Design review of the part built by this model. Coordinates are the model's own, in mm. A direction names the side the tool comes from. Coordinates: 2 decimals unless noted, no trailing zeros. Write each loop counter-clockwise with the first axis right and the second up, starting at its lowest first coordinate (ties: lowest second). Pieces come first, ordered by that corner, then holes.
```python
from build123d import *

# Parameters (mm, degrees)
SKETCH_1_R           = 23
EXTRUDE_1_DEPTH      = 26
SKETCH_7_R           = 23
SKETCH_7_R_2         = 15
CUT_EXTRUDE_5_DEPTH  = 8
SKETCH_8_R           = 9.5
CUT_EXTRUDE_6_DEPTH  = 6
SKETCH_9_R           = 3
CUT_EXTRUDE_7_DEPTH  = 24.5
SKETCH_10_R          = 20
CUT_EXTRUDE_8_DEPTH  = 10
CUT_EXTRUDE_START    = -6
SKETCH_11_R          = 9.5
CUT_EXTRUDE_10_DEPTH = 6


with BuildPart() as part:
    # 스케치1 → 보스-돌출1 (new body)
    with BuildSketch(Plane(origin=(0, 0, 0), x_dir=(1, 0, 0), z_dir=(0, 1, 0))):
        with Locations(Location((0, 0, 0), (0, 0, 90))):
            Circle(SKETCH_1_R)
    extrude(amount=EXTRUDE_1_DEPTH)

    # 스케치7 → 컷-돌출5 (cut)
    with BuildSketch(Plane(origin=(0, 0, 0), x_dir=(-1, 0, 0), z_dir=(0, -1, 0))):
        with Locations(Location((0, 0, 0), (0, 0, 90))):
            Circle(SKETCH_7_R)
        with Locations(Location((0, 0, 0), (0, 0, 90))):
            Circle(SKETCH_7_R_2, mode=Mode.SUBTRACT)
    extrude(amount=-CUT_EXTRUDE_5_DEPTH, mode=Mode.SUBTRACT)

    # 스케치8 → 컷-돌출6 (cut)
    with BuildSketch(Plane.XZ):
        with Locations(Location((0, 0, 0), (0, 0, 270))):
            Circle(SKETCH_8_R)
    extrude(amount=-CUT_EXTRUDE_6_DEPTH, mode=Mode.SUBTRACT)

    # 스케치9 → 컷-돌출7 (cut)
    with BuildSketch(Plane(origin=(0, 26, 0), x_dir=(1, 0, 0), z_dir=(0, 1, 0))):
        with Locations(Location((0, 0, 0), (0, 0, 270))):
            Circle(SKETCH_9_R)
    extrude(amount=-CUT_EXTRUDE_7_DEPTH, mode=Mode.SUBTRACT)

    # 스케치10 → 컷-돌출8 (cut)
    with BuildSketch(Plane(origin=(0, 26, 0), x_dir=(1, 0, 0), z_dir=(0, 1, 0))):
        with Locations(Location((0, 0, 0), (0, 0, 270))):
            Circle(SKETCH_10_R)
    extrude(amount=-CUT_EXTRUDE_8_DEPTH, mode=Mode.SUBTRACT)

    # 스케치11 → 컷-돌출10 (cut)
    with BuildSketch(Plane(origin=(0, 16, 0), x_dir=(1, 0, 0), z_dir=(0, 1, 0)).offset(CUT_EXTRUDE_START)):
        with Locations(Location((0, 0, 0), (0, 0, 90))):
            Circle(SKETCH_11_R)
    extrude(amount=CUT_EXTRUDE_10_DEPTH, mode=Mode.SUBTRACT)


solid = part.part
```
(1) Consider section B-B (z = 0). Give the boundary of the cut face in (x, y), plus the area to 3 significant figures.
(2) Mouldability with a two-part tool opening along Z and no side actions: class faces 1 (the flat face through (-19, 26, 7)), 2 (the cylindrical face through (0.66, 3.944, 14.985)), 3 (the flat face through (-4, 16, 9)) as +Z half, -Z half, draft (parallel to the pull), parting line (faces both ways), or undercut.
(3) Wall thickness on line 1 (X direction, y = 23.75, z = 0); line 2 (X direction, y = 13.7, z = 0); line 3 (Z direction, x = -0.5, y = 16.25): over which ranges is each line inside the solid? List them lowest first.
(4) Consider section D-D (x = -10.5). Give the boundary of the cut face in (y, z).
(5) For faces 4 (the cylindrical face through (5.78, 12.96, 7.54)), 5 (the flat face through (2.24, 6, 2.24)), 6 (the flat face through (0, 0, -10)), list the 3-axis set-ups (+Z, -Z, +X, -X, +Y, -Y) from which the entire face can be reached by the end or side of a thin tool; tool diameter is ignored.
(6) Insertion check: pin 1 Ø11.5 at (x, z) = (0, 0) entering from -Y; pin 2 Ø6 at (x, y) = (9, 5.5) entering from +Z; pin 3 Ø20 at (x, z) = (7, -5.5) entering from +Y. Each pin has a flat end and moves straight along its axis. Give the tip position at first contact, or say it passes through.
(7) Consider section A-A (x = 0). Give the boundary of the cut face in (y, z).
(8) Consider section C-C (z = -11.5). Give the boundary of the cut face in (x, y).
Results:
1. outline: (-23, 8) - (-15, 8) - (-15, 0) - (-9.5, 0) - (-9.5, 6) - (-3, 6) - (-3, 10) - (-9.5, 10) - (-9.5, 16) - (-20, 16) - (-20, 26) - (-23, 26) - close; (3, 6) - (9.5, 6) - (9.5, 0) - (15, 0) - (15, 8) - (23, 8) - (23, 26) - (20, 26) - (20, 16) - (9.5, 16) - (9.5, 10) - (3, 10) - close
1. area: 416 mm2
2. face 1: draft
2. face 2: parting line
2. face 3: undercut
3. line 1: x = -23 to -20, 20 to 23
3. line 2: x = -23 to -9.5, 9.5 to 23
3. line 3: z = -22.99 to -19.99, 19.99 to 22.99
4. outline: (0, -10.71) - (8, -10.71) - (8, -20.46) - (26, -20.46) - (26, -17.02) - (16, -17.02) - (16, 17.02) - (26, 17.02) - (26, 20.46) - (8, 20.46) - (8, 10.71) - (0, 10.71) - close
5. face 4: +Y
5. face 5: -Y
5. face 6: +Z, -Z, +X, -X, -Y
6. pin 1: stops at y = 6
6. pin 2: stops at z = 21.8
6. pin 3: stops at y = 16
7. outline: (0, -15) - (8, -15) - (8, -23) - (26, -23) - (26, -20) - (16, -20) - (16, -9.5) - (10, -9.5) - (10, -3) - (6, -3) - (6, -9.5) - (0, -9.5) - close; (0, 9.5) - (6, 9.5) - (6, 3) - (10, 3) - (10, 9.5) - (16, 9.5) - (16, 20) - (26, 20) - (26, 23) - (8, 23) - (8, 15) - (0, 15) - close
8. outline: (-19.92, 8) - (-9.63, 8) - (-9.63, 0) - (9.63, 0) - (9.63, 8) - (19.92, 8) - (19.92, 26) - (16.36, 26) - (16.36, 16) - (-16.36, 16) - (-16.36, 26) - (-19.92, 26) - close
